```python
from build123d import *

# Parameters (mm, degrees)
SKETCH_1_R          = 1.5
EXTRUDE_1_DEPTH     = 3
FILLET_1_R          = 10
SKETCH_2_R          = 1.5
CUT_EXTRUDE_1_DEPTH = 10


with BuildPart() as part:
    # 草圖1 → 填料-伸長1 (new body)
    with BuildSketch(Plane.XY):
        Polygon((80, 0), (80, 30), (0, 30), (0, 150), (80, 150), (80, 180), (160, 180), (160, 150), (240, 150), (240, 30), (160, 30), (160, 0), align=None)
        with Locations((15.5, 61.5)):
            Circle(SKETCH_1_R, mode=Mode.SUBTRACT)
        with Locations((44.5, 61.5)):
            Circle(SKETCH_1_R, mode=Mode.SUBTRACT)
        with Locations((44.5, 38.5)):
            Circle(SKETCH_1_R, mode=Mode.SUBTRACT)
        with Locations((15.5, 38.5)):
            Circle(SKETCH_1_R, mode=Mode.SUBTRACT)
        with Locations((44.5, 141.5)):
            Circle(SKETCH_1_R, mode=Mode.SUBTRACT)
        with Locations((15.5, 141.5)):
            Circle(SKETCH_1_R, mode=Mode.SUBTRACT)
        with Locations((15.5, 118.5)):
            Circle(SKETCH_1_R, mode=Mode.SUBTRACT)
        with Locations((44.5, 118.5)):
            Circle(SKETCH_1_R, mode=Mode.SUBTRACT)
        with Locations((35, 86.5)):
            Circle(SKETCH_1_R, mode=Mode.SUBTRACT)
        with Locations((25, 86.5)):
            Circle(SKETCH_1_R, mode=Mode.SUBTRACT)
        with Locations((60, 50)):
            Circle(SKETCH_1_R, mode=Mode.SUBTRACT)
        with Locations((25, 93.5)):
            Circle(SKETCH_1_R, mode=Mode.SUBTRACT)
        with Locations((35, 93.5)):
            Circle(SKETCH_1_R, mode=Mode.SUBTRACT)
        with Locations((60, 130)):
            Circle(SKETCH_1_R, mode=Mode.SUBTRACT)
        with Locations((180, 130)):
            Circle(SKETCH_1_R, mode=Mode.SUBTRACT)
        with Locations((205, 93.5)):
            Circle(SKETCH_1_R, mode=Mode.SUBTRACT)
        with Locations((215, 93.5)):
            Circle(SKETCH_1_R, mode=Mode.SUBTRACT)
        with Locations((180, 50)):
            Circle(SKETCH_1_R, mode=Mode.SUBTRACT)
        with Locations((215, 86.5)):
            Circle(SKETCH_1_R, mode=Mode.SUBTRACT)
        with Locations((205, 86.5)):
            Circle(SKETCH_1_R, mode=Mode.SUBTRACT)
        with Locations((195.5, 118.5)):
            Circle(SKETCH_1_R, mode=Mode.SUBTRACT)
        with Locations((224.5, 118.5)):
            Circle(SKETCH_1_R, mode=Mode.SUBTRACT)
        with Locations((224.5, 141.5)):
            Circle(SKETCH_1_R, mode=Mode.SUBTRACT)
        with Locations((195.5, 141.5)):
            Circle(SKETCH_1_R, mode=Mode.SUBTRACT)
        with Locations((224.5, 38.5)):
            Circle(SKETCH_1_R, mode=Mode.SUBTRACT)
        with Locations((195.5, 38.5)):
            Circle(SKETCH_1_R, mode=Mode.SUBTRACT)
        with Locations((195.5, 61.5)):
            Circle(SKETCH_1_R, mode=Mode.SUBTRACT)
        with Locations((224.5, 61.5)):
            Circle(SKETCH_1_R, mode=Mode.SUBTRACT)
    extrude(amount=EXTRUDE_1_DEPTH)

    # 圓角1
    fillet_1_edges = [part.edges().sort_by_distance(p)[0] for p in [
        (80, 0, 1.5),
        (80, 30, 1.5),
        (0, 30, 1.5),
        (0, 150, 1.5),
        (80, 150, 1.5),
        (80, 180, 1.5),
        (160, 180, 1.5),
        (160, 150, 1.5),
        (240, 150, 1.5),
        (240, 30, 1.5),
        (160, 30, 1.5),
        (160, 0, 1.5),
    ]]
    fillet(fillet_1_edges, radius=FILLET_1_R)

    # 草圖2 → 除料-伸長1 (cut)
    with BuildSketch(Plane.XY.offset(3)):
        with Locations((231.801662433, 85.38)):
            Circle(SKETCH_2_R)
        with Locations((231.7, 33.38)):
            Circle(SKETCH_2_R)
    extrude(amount=-CUT_EXTRUDE_1_DEPTH, mode=Mode.SUBTRACT)


solid = part.part
```
Verification items for the finished model (mm, model axes). Coordinates: 2 decimals unless noted, no trailing zeros. Order: outer loops, then holes, each group sorted by start corner. A loop starts at its lowest first (then second) coordinate and runs counter-clockwise, first axis right, second up. Notation, with made-up numbers: (-37, -36.75) - (7, -36.75) arc R8 ccw to (7, -22.75) - close; hole circle Ø8 at (-33.5, 28.25). An arc over 180 degrees is marked (long way). Return JSON: item names as keys, results as strings.
(1) Section check A-A, the plane z = 1.35. Give the number of separate pieces and of enclosed holes in the cut face, and give its area (3 significant figures).
Filled sheet:
{"separate pieces": "1", "enclosed holes": "30", "area": "33,300 mm^2"}
(2) Thickness scan on line 1 along X through (y, z) = (118.5, 0.9); line 2 along Y through (x, z) = (215, 1.8); line 3 along X through (y, z) = (141.5, 0.9). Record the ranges inside material, lowest first.
Filled sheet:
{"line 1": "x = 0 to 14, 17 to 43, 46 to 194, 197 to 223, 226 to 240", "line 2": "y = 30 to 85, 88 to 92, 95 to 150", "line 3": "x = 0.11 to 14, 17 to 43, 46 to 194, 197 to 223, 226 to 239.89"}
(3) Section check B-B, the plane x = 157. Record the cut outline in (y, z), and give its area (3 significant figures).
Filled sheet:
{"outline": "(2.86, 0) - (177.14, 0) - (177.14, 3) - (2.86, 3) - close", "area": "523 mm^2"}
(4) Go/stop test with flat-tipped pins: pin 1 (1.8 mm diameter, centred on x = 25, y = 93.5, fed in from +Z); pin 2 (1 mm diameter, centred on x = 189.5, z = 2, fed in from -Y). Record where each tip stops, or that it passes through.
Filled sheet:
{"pin 1": "passes through", "pin 2": "stops at y = 30"}
